Could you check a few things on this drawing? It's one solid part, dimensions in mm from its lowest x, y, z. Give positions to 0.01 mm unless a question says otherwise; leave off trailing zeros. Write each loop counter-clockwise with the first axis right and the second up, starting at its lowest first coordinate (ties: lowest second). Pieces come first, ordered by that corner, then holes. Notation, with made-up numbers: M 48,-33.5 L 74,-33.5 A16 ccw 74,-9.5 Z; hole C 16.25,56.5 d7. An arc over 180 degrees is marked long. Answer as CSV lines item,"result". Start each with the question number.
Q1. If I drill on line 1 along Y through (x, z) = (20, 115.5); line 2 along X through (y, z) = (42, 71.5); line 3 along X through (y, z) = (43.5, 46.5), over which ranges is the centre line in solid material (lowest first)?
Q2. Suppose I cut it at A-A (x = 20). Write out the boundary of the cut face in (y, z), then the cut area to 3 significant figures.
Q3. Suppose I cut it at C-C (z = 26.5). Write out the boundary of the cut face in (x, y).
Q4. Thinking about a two-plate mould opening in Y: for the marked faces 1, 2 and 3, which applies, +Y half, -Y half, draft (parallel to the pull), parting line (faces both ways), or undercut?
Q5. For pin 1 (12 mm diameter, centred on x = 20, y = 40, fed in from +Z); pin 2 (4 mm diameter, centred on y = 21.5, z = 66, fed in from -X), each with a flat end and sliding along its axis, tell me the tip position at first contact or that it passes through.
Q6. Suppose I cut it at B-B (y = 40). Write out the boundary of the cut face in (x, z).
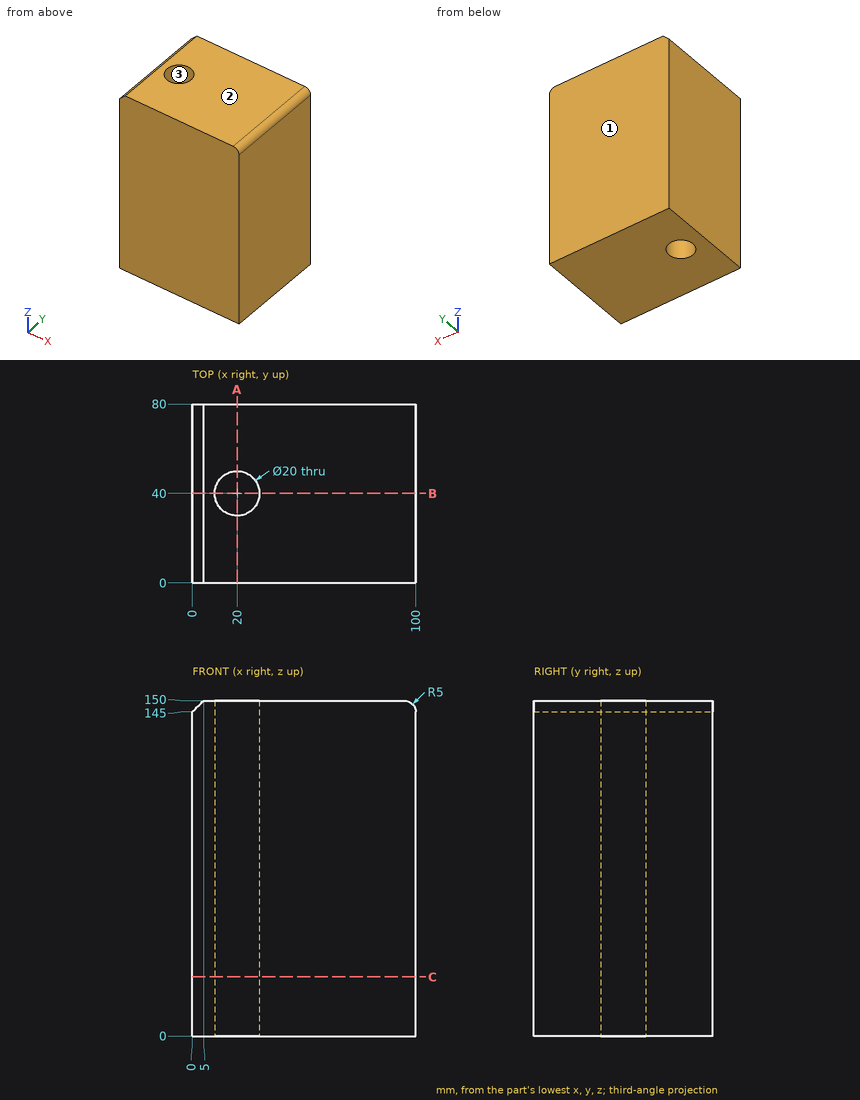
Resolved:
1,line 1,"0 to 30, 50 to 80"
1,line 2,"0 to 10.2, 29.8 to 100"
1,line 3,"0 to 10.63, 29.37 to 100"
2,outline,"M 0,0 L 30,0 L 30,150 L 0,150 Z; M 50,0 L 80,0 L 80,150 L 50,150 Z"
2,area,"9,000 mm^2"
3,outline,"M 0,0 L 100,0 L 100,80 L 0,80 Z; hole C 20,40 d20"
4,face 1,"+Y half"
4,face 2,"draft"
4,face 3,"undercut"
5,pin 1,"through"
5,pin 2,"x = 0"
6,outline,"M 0,0 L 10,0 L 10,150 L 5,150 L 0,145 Z; M 30,0 L 100,0 L 100,145 A5 ccw 95,150 L 30,150 Z"
